```python
from build123d import *

# Parameters (mm, degrees)
SKETCH1_R           = 8.5
SKETCH1_R_2         = 3
BOSS_EXTRUDE1_DEPTH = 6
SKETCH2_R           = 7.5
SKETCH2_R_2         = 4.5
CUT_EXTRUDE1_DEPTH  = 0.1
CUT_EXTRUDE2_START  = -0.1
SKETCH3_R           = 7.5
SKETCH3_R_2         = 4.5
CUT_EXTRUDE2_DEPTH  = 0.1
FILLET1_R           = 0.2


with BuildPart() as part:
    # Sketch1 → Boss-Extrude1 (new body)
    with BuildSketch(Plane(origin=(0, 0, 0), x_dir=(0, 0, -1), z_dir=(1, 0, 0))):
        Circle(SKETCH1_R)
        Circle(SKETCH1_R_2, mode=Mode.SUBTRACT)
    extrude(amount=BOSS_EXTRUDE1_DEPTH)

    # Sketch2 → Cut-Extrude1 (cut)
    with BuildSketch(Plane(origin=(6, 0, 0), x_dir=(0, 0, -1), z_dir=(1, 0, 0))):
        Circle(SKETCH2_R)
        Circle(SKETCH2_R_2, mode=Mode.SUBTRACT)
    extrude(amount=-CUT_EXTRUDE1_DEPTH, mode=Mode.SUBTRACT)

    # Sketch3 → Cut-Extrude2 (cut)
    with BuildSketch(Plane.ZY.offset(CUT_EXTRUDE2_START)):
        with Locations(Location((0, 0, 0), (0, 0, 180))):
            Circle(SKETCH3_R)
        with Locations(Location((0, 0, 0), (0, 0, 180))):
            Circle(SKETCH3_R_2, mode=Mode.SUBTRACT)
    extrude(amount=CUT_EXTRUDE2_DEPTH, mode=Mode.SUBTRACT)

    # Fillet1
    fillet1_edges = [part.edges().sort_by_distance(p)[0] for p in [
        (0, 0, 8.5),
        (6, 0, 8.5),
        (0, 0, 3),
        (6, 0, 3),
    ]]
    fillet(fillet1_edges, radius=FILLET1_R)


solid = part.part
```
Verification items for the finished model (mm, model axes). A direction names the side the tool comes from. Give positions to 0.01 mm unless a question says otherwise; leave off trailing zeros. Loops run counter-clockwise (first coordinate to the right, second up) from the corner with the lowest first, then second, coordinate; pieces in that order, holes last. Notation, with made-up numbers: M -17,74.25 L -11,74.25 A33 cw -11,103.25 Z; hole C 82.5,-36.75 d4. An arc over 180 degrees is marked long. One line per question, with ' | ' between items.
Item 1: Thickness scan on line 1 (Y direction, x = 0.05, z = 0); line 2 (X direction, y = 3.75, z = -4.5); line 3 (Y direction, x = 0.5, z = -2.5). Record the ranges inside material, lowest first. Write a range as [from, to].
Completed:
line 1: y = [-8.43, -7.5], [-4.5, -3.07], [3.07, 4.5], [7.5, 8.43] | line 2: x = [0.1, 5.9] | line 3: y = [-8.12, -1.66], [1.66, 8.12]
Item 2: Draft check along Y on faces 1 (the face through (6, -7, 4)), 2 (the face through (2.961, 7.167, -4.57)), 3 (the face through (3, 0, 3)). Enter one of: +Y half, -Y half, draft (parallel to the pull), parting line (faces both ways), or undercut.
Completed:
face 1: draft | face 2: parting line | face 3: undercut
Item 3: Depth check by flat-ended pin: P1, Ø8, axis at y = 0, z = 0, coming from the +X side; P2, Ø1, axis at x = 2, z = -3, coming from the -Y side; P3, Ø2, axis at x = 3, y = -6, coming from the +Z side. Enter the tip coordinate at first touch or a pass-through.
Completed:
P1: stops at x = 6 | P2: stops at y = -8.12 | P3: stops at z = 6.87
Item 4: Section check C-C, the plane x = 2.6. Record the cut outline in (y, z), plus the area to 3 significant figures.
Completed:
outline: C 0,0 d17; hole C 0,0 d6 | area: 199 mm^2
Item 5: Tool access check on faces 4 (the face through (0.1, 5, 0)), 5 (the face through (5.9, -5, 0)), 6 (the face through (0, -3, -2)). Record the directions out of +Z, -Z, +X, -X, +Y, -Y that give a thin tool (end or side, any length) a straight path to the whole face; none if there is none.
Completed:
face 4: -X | face 5: +X | face 6: +Z, -Z, -X, +Y, -Y
